from build123d import *

# Parameters (mm, degrees)
SKETCH_1_W          = 30
SKETCH_1_H          = 42.5
EXTRUDE_1_DEPTH     = 40
SKETCH_2_W          = 25.29109927
SKETCH_2_H          = 38.153739886
CUT_EXTRUDE_1_DEPTH = 20
SKETCH_3_R          = 10
CUT_EXTRUDE_2_DEPTH = 1
SKETCH_4_W          = 41
SKETCH_4_H          = 42.5
SKETCH_4_R          = 1
EXTRUDE_2_DEPTH     = 5


with BuildPart() as part:
    # 草图1 → 凸台-拉伸1 (new body)
    with BuildSketch(Plane.XY):
        Rectangle(SKETCH_1_W, SKETCH_1_H)
    extrude(amount=EXTRUDE_1_DEPTH)

    # 草图2 → 切除-拉伸1 (cut)
    with BuildSketch(Plane.XY.offset(40)):
        Rectangle(SKETCH_2_W, SKETCH_2_H)
    extrude(amount=-CUT_EXTRUDE_1_DEPTH, mode=Mode.SUBTRACT)

    # 草图3 → 切除-拉伸2 (cut)
    with BuildSketch(Plane(origin=(0, 0, 0), x_dir=(-1, 0, 0), z_dir=(0, 0, -1))):
        Circle(SKETCH_3_R)
    extrude(amount=-CUT_EXTRUDE_2_DEPTH, mode=Mode.SUBTRACT)

    # 草图4 → 凸台-拉伸2 (add)
    with BuildSketch(Plane(origin=(0, 0, 0), x_dir=(-1, 0, 0), z_dir=(0, 0, -1))):
        Rectangle(SKETCH_4_W, SKETCH_4_H)
        with Locations((17.9, 8.65)):
            Circle(SKETCH_4_R, mode=Mode.SUBTRACT)
        with Locations(Location((-17.9, 8.65, 0), (0, 0, 180))):
            Circle(SKETCH_4_R, mode=Mode.SUBTRACT)
        with Locations((-17.9, -8.65)):
            Circle(SKETCH_4_R, mode=Mode.SUBTRACT)
        with Locations(Location((17.9, -8.65, 0), (0, 0, 180))):
            Circle(SKETCH_4_R, mode=Mode.SUBTRACT)
    extrude(amount=EXTRUDE_2_DEPTH)


solid = part.part
Source: CAD feature listing. Evaluate the final solid. Frame: model axes, mm. A direction names the side the tool comes from. Round coordinates to 2 decimals unless told otherwise and drop trailing zeros. Order: outer loops, then holes, each group sorted by start corner. A loop starts at its lowest first (then second) coordinate and runs counter-clockwise, first axis right, second up. Notation, with made-up numbers: (72, 6.25) - (108, 6.25) arc R30 ccw to (108, 31.25) - close; hole circle Ø11 at (22, 61). An arc over 180 degrees is marked (long way). Use a Markdown table: item, result. Add a question column.
1. First-contact query: pin 1 (22 mm diameter, centred on y = -7, z = 32, fed in from +X); pin 2 (6 mm diameter, centred on y = 2.5, z = 31.5, fed in from -X); pin 3 (1.6 mm diameter, centred on x = -18.5, y = -6, fed in from +Z); pin 4 (6 mm diameter, centred on x = 17, y = -7, fed in from +Z). Flat tips, straight axial feed; report the tip coordinate or a pass-through.
2. Line query: probe 1 along Y at (x, z) = (17.9, -1.5); probe 2 along X at (y, z) = (16.5, 32); probe 3 along Y at (x, z) = (1, 33). Output: solid intervals per line, ascending.
3. Set-up query: faces 4 (the flat face through (0, 0, 1)), 5 (the flat face through (18, 0, 0)), 6 (the flat face through (0, -19.077, 30)). Return all of +Z, -Z, +X, -X, +Y, -Y with unobstructed straight access to the full face (end or side cutting, diameter ignored); none if empty.
4. Section query A-A (x = 0). Return the cut outline in (y, z).
5. Mould query, pull axis Y, two halves, no side actions, for faces 1 (the flat face through (0, 0, -5)), 2 (the flat face through (-12.646, 0, 30)), 3 (the flat face through (0, -21.25, 18)). Classes: +Y half, -Y half, draft (parallel to the pull), parting line (faces both ways), or undercut.
6. Section query C-C (y = 8.65). Return the cut outline in (x, z).
7. Section query D-D (z = 32). Return the cut outline in (x, y).
8. Section query B-B (y = 0). Return the cut outline in (x, z).
Derived:
| question | item | result |
|---|---|---|
| 1 | pin 1 | x = 15 |
| 1 | pin 2 | x = -15 |
| 1 | pin 3 | z = 0 |
| 1 | pin 4 | z = 40 |
| 2 | probe 1 | -21.25 to -9.65, -7.65 to 7.65, 9.65 to 21.25 |
| 2 | probe 2 | -15 to -12.65, 12.65 to 15 |
| 2 | probe 3 | -21.25 to -19.08, 19.08 to 21.25 |
| 3 | face 4 | none |
| 3 | face 5 | +Z, +X, +Y, -Y |
| 3 | face 6 | +Z |
| 4 | outline | (-21.25, -5) - (21.25, -5) - (21.25, 40) - (19.08, 40) - (19.08, 20) - (-19.08, 20) - (-19.08, 40) - (-21.25, 40) - close; hole (-10, 0) - (10, 0) - (10, 1) - (-10, 1) - close |
| 5 | face 1 | draft |
| 5 | face 2 | undercut |
| 5 | face 3 | -Y half |
| 6 | outline | (-20.5, -5) - (-18.9, -5) - (-18.9, 0) - (-20.5, 0) - close; (-16.9, -5) - (16.9, -5) - (16.9, 0) - (15, 0) - (15, 40) - (12.65, 40) - (12.65, 20) - (-12.65, 20) - (-12.65, 40) - (-15, 40) - (-15, 0) - (-16.9, 0) - close; (18.9, -5) - (20.5, -5) - (20.5, 0) - (18.9, 0) - close; hole (-5.02, 0) - (5.02, 0) - (5.02, 1) - (-5.02, 1) - close |
| 7 | outline | (-15, -21.25) - (15, -21.25) - (15, 21.25) - (-15, 21.25) - close; hole (-12.65, -19.08) - (12.65, -19.08) - (12.65, 19.08) - (-12.65, 19.08) - close |
| 8 | outline | (-20.5, -5) - (20.5, -5) - (20.5, 0) - (15, 0) - (15, 40) - (12.65, 40) - (12.65, 20) - (-12.65, 20) - (-12.65, 40) - (-15, 40) - (-15, 0) - (-20.5, 0) - close; hole (-10, 0) - (10, 0) - (10, 1) - (-10, 1) - close |
